```python
from build123d import *

# Parameters (mm, degrees)
SKETCH1_W           = 43.18
SKETCH1_H           = 50.8
SKETCH1_R           = 1.524
SKETCH1_R_2         = 3.175
SKETCH1_R_3         = 12.7
BOSS_EXTRUDE1_DEPTH = 6.35
CHAMFER1_SIZE       = 0.254


with BuildPart() as part:
    # Sketch1 → Boss-Extrude1 (new body)
    with BuildSketch(Plane.XY):
        Rectangle(SKETCH1_W, SKETCH1_H)
        with Locations((-15.494, 15.494)):
            Circle(SKETCH1_R, mode=Mode.SUBTRACT)
        with Locations((-9.525, 15.875)):
            Circle(SKETCH1_R_2, mode=Mode.SUBTRACT)
        with Locations((-15.494, -15.494)):
            Circle(SKETCH1_R, mode=Mode.SUBTRACT)
        with Locations((-9.525, -15.875)):
            Circle(SKETCH1_R_2, mode=Mode.SUBTRACT)
        with Locations((9.525, -15.875)):
            Circle(SKETCH1_R_2, mode=Mode.SUBTRACT)
        with Locations((15.494, -15.494)):
            Circle(SKETCH1_R, mode=Mode.SUBTRACT)
        with Locations((9.525, 15.875)):
            Circle(SKETCH1_R_2, mode=Mode.SUBTRACT)
        with Locations((15.494, 15.494)):
            Circle(SKETCH1_R, mode=Mode.SUBTRACT)
        Circle(SKETCH1_R_3, mode=Mode.SUBTRACT)
    extrude(amount=BOSS_EXTRUDE1_DEPTH)

    # Chamfer1
    chamfer1_edges = [part.edges().sort_by_distance(p)[0] for p in [
        (-21.59, 0, 6.35),
        (-17.018, 15.494, 0),
        (-17.018, 15.494, 6.35),
        (0, -25.4, 6.35),
        (-12.7, 15.875, 0),
        (-12.7, 15.875, 6.35),
        (-17.018, -15.494, 0),
        (-17.018, -15.494, 6.35),
        (-12.7, -15.875, 0),
        (-12.7, -15.875, 6.35),
        (6.35, -15.875, 0),
        (6.35, -15.875, 6.35),
        (13.97, -15.494, 0),
        (13.97, -15.494, 6.35),
        (6.35, 15.875, 0),
        (6.35, 15.875, 6.35),
        (13.97, 15.494, 0),
        (13.97, 15.494, 6.35),
        (21.59, 0, 6.35),
        (-12.7, 0, 0),
        (-12.7, 0, 6.35),
        (0, -25.4, 0),
        (-21.59, 0, 0),
        (0, 25.4, 0),
        (21.59, 0, 0),
        (0, 25.4, 6.35),
    ]]
    chamfer(chamfer1_edges, length=CHAMFER1_SIZE)


solid = part.part
```
Input: part model. Units: mm. Frame: model coordinates. Coordinates: 2 decimals unless noted, no trailing zeros. Write each loop counter-clockwise with the first axis right and the second up, starting at its lowest first coordinate (ties: lowest second). Pieces come first, ordered by that corner, then holes.
1) Section C-C on z = 5.5. State how many separate pieces and enclosed holes the cut face has, and give its area (3 significant figures).
2) Pin query (flat end, axial travel): pin 1 Ø3.5 at (x, y) = (-15.494, 15.494) entering from +Z; pin 2 Ø23 at (x, y) = (0, 0) entering from -Z. Return the tip coordinate at first contact, or that it passes through.
3) Mould query, pull axis X, two halves, no side actions, for faces 1 (the cylindrical face through (-12.697, 16.015, 3.134)), 2 (the flat face through (0, 25.4, 3)). Classes: pulls with the +X half, pulls with the -X half, needs draft (parallel to the pull), parting line crosses it, or undercut.
4) Section B-B on y = 0. Output: boundary loops of the cut face in (x, z), and give its area (3 significant figures).
5) Section A-A on x = 0. Output: boundary loops of the cut face in (y, z).
6) Material intervals for line 1 along Y through (x, z) = (0, 1.55); line 2 along X through (y, z) = (-11, 3.25); line 3 along X through (y, z) = (18, 1), sorted ascending.
Check result:
1. separate pieces: 1
1. enclosed holes: 9
1. area: 1,530 mm2
2. pin 1: stops at z = 6.32
2. pin 2: passes through
3. face 1: undercut
3. face 2: needs draft
4. outline: (-21.59, 0.25) - (-21.34, 0) - (-12.95, 0) - (-12.7, 0.25) - (-12.7, 6.1) - (-12.95, 6.35) - (-21.34, 6.35) - (-21.59, 6.1) - close; (12.7, 0.25) - (12.95, 0) - (21.34, 0) - (21.59, 0.25) - (21.59, 6.1) - (21.34, 6.35) - (12.95, 6.35) - (12.7, 6.1) - close
4. area: 113 mm2
5. outline: (-25.4, 0.25) - (-25.15, 0) - (-12.95, 0) - (-12.7, 0.25) - (-12.7, 6.1) - (-12.95, 6.35) - (-25.15, 6.35) - (-25.4, 6.1) - close; (12.7, 0.25) - (12.95, 0) - (25.15, 0) - (25.4, 0.25) - (25.4, 6.1) - (25.15, 6.35) - (12.95, 6.35) - (12.7, 6.1) - close
6. line 1: y = -25.4 to -12.7, 12.7 to 25.4
6. line 2: x = -21.59 to -6.35, 6.35 to 21.59
6. line 3: x = -21.59 to -11.88, -7.17 to 7.17, 11.88 to 21.59
